Answer from the drawing. Dimensions are ordinates in mm from the lowest x, y and z of the part. Coordinates: 2 decimals unless noted, no trailing zeros. Order: outer loops, then holes, each group sorted by start corner. A loop starts at its lowest first (then second) coordinate and runs counter-clockwise, first axis right, second up. Notation, with made-up numbers: M -27.75,47.5 L 16.25,47.5 A16 cw 16.25,57.5 Z; hole C 59.5,-26.5 d9. An arc over 180 degrees is marked long. Use a Markdown table: item, result.
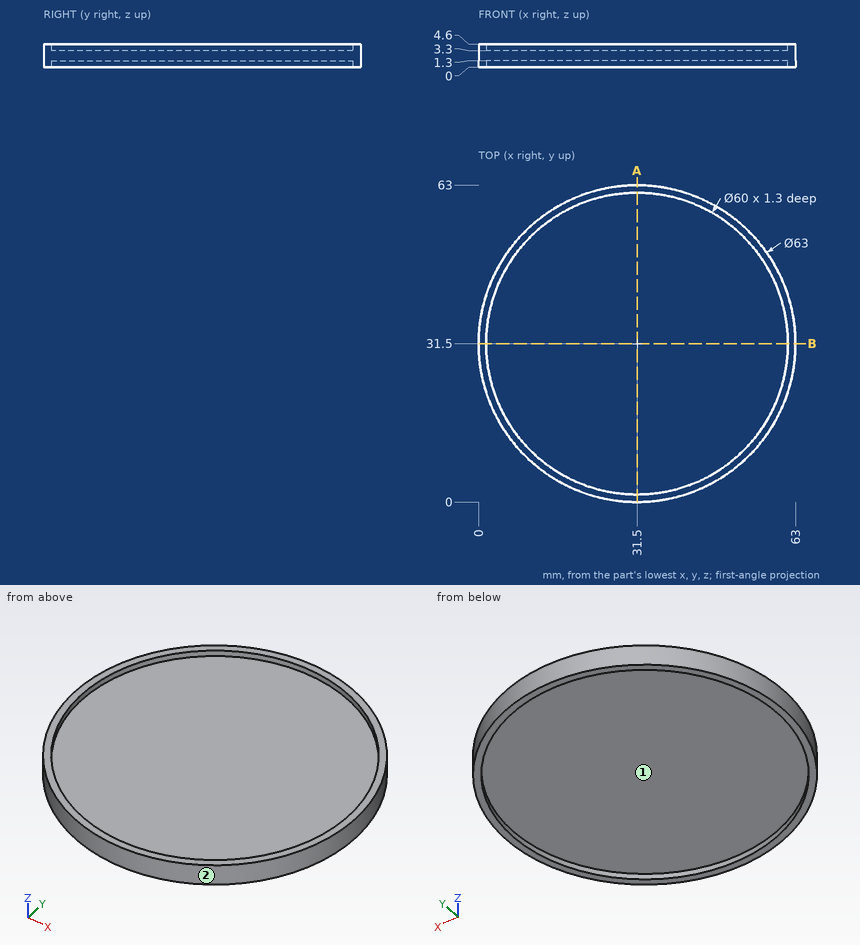
(1) Straight lines are drawn through the part: L1, parallel to Y at x = 31.5, z = 3.8; L2, parallel to Z at x = 40.5, y = 59.5; L3, parallel to X at y = 15, z = 0.65. For each, find the intervals that lie inside material, in ascending order.
Conclusion:
| item | result |
|---|---|
| L1 | 0 to 1.5, 61.5 to 63 |
| L2 | 1.3 to 3.3 |
| L3 | 4.67 to 6.45, 56.55 to 58.33 |
(2) Given P1, Ø4, axis at x = 56.5, y = 33, coming from the -Z side; P2, Ø2, axis at y = 25.5, z = 2.5, coming from the +X side; P3, Ø8, axis at x = 56, y = 26, coming from the +Z side, each flat-ended and moving along its own axis, determine where each tip first touches the part or whether it passes through.
Conclusion:
| item | result |
|---|---|
| P1 | z = 1.3 |
| P2 | x = 62.6 |
| P3 | z = 3.3 |
(3) Determine the mould class of the marked faces 1 and 2 for opening direction Y: pulls with the +Y half, pulls with the -Y half, needs draft (parallel to the pull), parting line crosses it, or undercut.
Conclusion:
| item | result |
|---|---|
| face 1 | undercut |
| face 2 | parting line crosses it |
(4) A cutting plane is placed at A-A (x = 31.5). Determine the outline of the cut face in (y, z).
Conclusion:
| item | result |
|---|---|
| outline | M 0,0 L 1.5,0 L 1.5,1.3 L 61.5,1.3 L 61.5,0 L 63,0 L 63,4.6 L 61.5,4.6 L 61.5,3.3 L 1.5,3.3 L 1.5,4.6 L 0,4.6 Z |
